Build history of the part. All positions in model axes, mm. Give positions to 0.01 mm unless a question says otherwise; leave off trailing zeros. Order: outer loops, then holes, each group sorted by start corner. A loop starts at its lowest first (then second) coordinate and runs counter-clockwise, first axis right, second up. Notation, with made-up numbers: (-33.5, 76.25) - (18.5, 76.25) arc R20 ccw to (18.5, 85.25) - close; hole circle Ø7 at (28, 52.5). An arc over 180 degrees is marked (long way). Write each question's results on one line, items separated by ' | '. Start each with the question number.
1) Cut at B-B on z = 25.5. List the corners of the cut face in (x, y) (3 decimals).
2) Cut at C-C on y = 0.5. State how many separate pieces and enclosed holes the cut face has, plus the area to 3 significant figures.
3) Drill centre lines: line 1 along Z through (x, y) = (107.95, 1.5); line 2 along Z through (x, y) = (-38.1, 2); line 3 along X through (y, z) = (0.5, 41.5) (3 decimals). Where is each one in solid material? Low to high. Write a range as from..to.
4) Cut at A-A on x = -63. List the corners of the cut face in (y, z) (3 decimals), plus the area to 3 significant figures.
from build123d import *

# Parameters (mm, degrees)
SKETCH1_W                  = 298.45
SKETCH1_H                  = 495.3
BOSS_EXTRUDE1_DEPTH        = 3.175
CUT_EXTRUDE1_DEPTH         = 290.203986184
CUT_EXTRUDE1_DEPTH_BACK    = 290.203986184
SKETCH3_W                  = 196.85
SKETCH3_H                  = 114.3
F_12_CLEARANCE_HOLE2_D     = 5.6134
F_12_CLEARANCE_HOLE2_DEPTH = 16.51
F_12_CLEARANCE_HOLE2_TIP   = 1.686435499
SKETCH20_W                 = 47.879
SKETCH20_H                 = 47.879
CUT_EXTRUDE5_DEPTH         = 290.203986184
F_10_CLEARANCE_HOLE1_D     = 5.1054
F_10_CLEARANCE_HOLE1_DEPTH = 10.668
F_10_CLEARANCE_HOLE1_TIP   = 1.533816902


with BuildPart() as part:
    # Sketch1 → Boss-Extrude1 (new, symmetric)
    with BuildSketch(Plane(origin=(0, 0, 0), x_dir=(1, 0, 0), z_dir=(0, 1, 0))):
        Rectangle(SKETCH1_W, SKETCH1_H)
    extrude(amount=BOSS_EXTRUDE1_DEPTH, both=True)

    # Sketch3 → Cut-Extrude1 (cut, two sides: drawn at the far end of the back side and taken through both)
    with BuildSketch(Plane(origin=(0, 3.175, 0), x_dir=(1, 0, 0), z_dir=(0, 1, 0)).offset(-CUT_EXTRUDE1_DEPTH_BACK)):
        with Locations((0, -44.45)):
            Rectangle(SKETCH3_W, SKETCH3_H)
    extrude(amount=CUT_EXTRUDE1_DEPTH + CUT_EXTRUDE1_DEPTH_BACK, mode=Mode.SUBTRACT)

    # #12 Clearance Hole2
    with Locations(Plane(origin=(0, -3.175, 0), x_dir=(-1, 0, 0), z_dir=(0, -1, 0))):
        with Locations((107.95, -223.8375), (133.35, -223.8375), (133.35, 223.8375), (107.95, 223.8375), (-133.35, 223.8375), (-107.95, 223.8375), (-133.35, -223.8375), (-107.95, -223.8375)):
            Hole(F_12_CLEARANCE_HOLE2_D / 2, depth=F_12_CLEARANCE_HOLE2_DEPTH)
            with Locations((0, 0, -(F_12_CLEARANCE_HOLE2_DEPTH + F_12_CLEARANCE_HOLE2_TIP / 2))):  # 118° drill point
                Cone(0, F_12_CLEARANCE_HOLE2_D / 2, F_12_CLEARANCE_HOLE2_TIP, mode=Mode.SUBTRACT)

    # Sketch20 → Cut-Extrude5 (cut, through all)
    with BuildSketch(Plane.XZ.offset(3.175)):
        with Locations((0, 171.45)):
            Rectangle(SKETCH20_W, SKETCH20_H)
    extrude(amount=-CUT_EXTRUDE5_DEPTH, mode=Mode.SUBTRACT)

    # #10 Clearance Hole1
    with Locations(Plane(origin=(0, -3.175, 0), x_dir=(-1, 0, 0), z_dir=(0, -1, 0))):
        with Locations((-38.1, -155.575), (38.1, -155.575), (38.1, -187.325), (-38.1, -187.325)):
            Hole(F_10_CLEARANCE_HOLE1_D / 2, depth=F_10_CLEARANCE_HOLE1_DEPTH)
            with Locations((0, 0, -(F_10_CLEARANCE_HOLE1_DEPTH + F_10_CLEARANCE_HOLE1_TIP / 2))):  # 118° drill point
                Cone(0, F_10_CLEARANCE_HOLE1_D / 2, F_10_CLEARANCE_HOLE1_TIP, mode=Mode.SUBTRACT)


solid = part.part
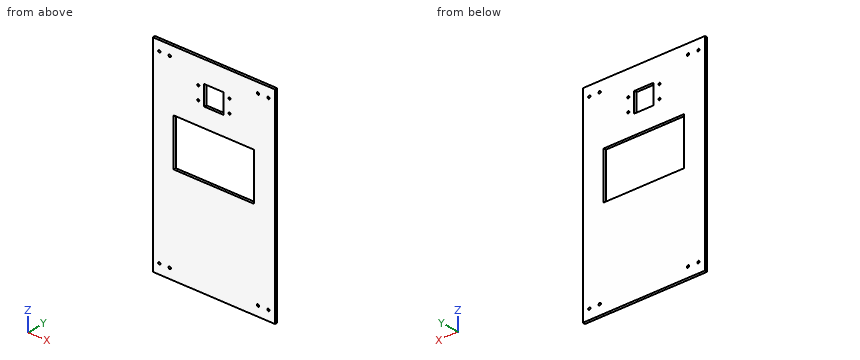
Results:
1) outline: (-149.225, -3.175) - (-98.425, -3.175) - (-98.425, 3.175) - (-149.225, 3.175) - close; (98.425, -3.175) - (149.225, -3.175) - (149.225, 3.175) - (98.425, 3.175) - close
2) separate pieces: 1 | enclosed holes: 14 | area: 123,000 mm^2
3) line 1: -247.65..-226.64, -221.03..221.03, 226.64..247.65 | line 2: -247.65..-12.7, 101.6..153.02, 158.13..184.77, 189.88..247.65 | line 3: -149.225..-98.425, 98.425..149.225
4) outline: (-3.175, -247.65) - (3.175, -247.65) - (3.175, -12.7) - (-3.175, -12.7) - close; (-3.175, 101.6) - (3.175, 101.6) - (3.175, 247.65) - (-3.175, 247.65) - close | area: 2,420 mm^2
